Build history of the part. All positions in model axes, mm. Face numbers are marked on the shaded views. A direction names the side the tool comes from. Give positions to 0.01 mm unless a question says otherwise; leave off trailing zeros. Order: outer loops, then holes, each group sorted by start corner. A loop starts at its lowest first (then second) coordinate and runs counter-clockwise, first axis right, second up. Notation, with made-up numbers: (60, 41) - (69, 41) arc R18 cw to (69, 63) - close; hole circle Ø4 at (-25.5, 18.5). An arc over 180 degrees is marked (long way). Use a Markdown table: item, result.
from build123d import *

# Parameters (mm, degrees)
CROQUIS2_R              = 1.55
SALIENTE_EXTRUIR1_DEPTH = 5
REDONDEO9_R             = 5


with BuildPart() as part:
    # Croquis2 → Saliente-Extruir1 (new body)
    with BuildSketch(Plane(origin=(0, 0, 0), x_dir=(1, 0, 0), z_dir=(0, 1, 0))):
        Polygon((16, -17.5), (16, 17.5), (-16, 17.5), (-16, 8), (12, 8), (12, -8), (-16, -8), (-16, -17.5), align=None)
        with Locations(Location((-12.5, -12.5, 0), (0, 0, 270))):
            Circle(CROQUIS2_R, mode=Mode.SUBTRACT)
        with Locations(Location((12.5, -12.5, 0), (0, 0, 270))):
            Circle(CROQUIS2_R, mode=Mode.SUBTRACT)
        with Locations(Location((-12.5, 12.5, 0), (0, 0, 270))):
            Circle(CROQUIS2_R, mode=Mode.SUBTRACT)
        with Locations(Location((12.5, 12.5, 0), (0, 0, 270))):
            Circle(CROQUIS2_R, mode=Mode.SUBTRACT)
    extrude(amount=SALIENTE_EXTRUIR1_DEPTH)

    # Redondeo9
    # the kernel refuses this fillet: 5 mm, written as the material it adds along each edge
    with BuildSketch(Plane(origin=(12, 0, 8), x_dir=(0, 0, -1), z_dir=(0, 1, 0)), Plane(origin=(12, 0, -8), x_dir=(-1, 0, 0), z_dir=(0, 1, 0))) as redondeo9_piece_1:
        with BuildLine():
            CenterArc((REDONDEO9_R, REDONDEO9_R), REDONDEO9_R, 180, 90)
            Line((0, REDONDEO9_R), (0, 0))
            Line((0, 0), (REDONDEO9_R, 0))
        make_face()
    extrude(amount=5)
    # the kernel refuses this fillet: 5 mm, written as the material it takes off along each edge
    with BuildSketch(Plane(origin=(-16, -12.5, 8), x_dir=(0, 0, 1), z_dir=(0, 1, 0))) as redondeo9_2_piece_1:
        with BuildLine():
            CenterArc((REDONDEO9_R, REDONDEO9_R), REDONDEO9_R, 180, 90)
            Line((0, REDONDEO9_R), (0, 0))
            Line((0, 0), (REDONDEO9_R, 0))
        make_face()
    extrude(amount=30, mode=Mode.SUBTRACT)
    with BuildSketch(Plane(origin=(-16, -12.5, 17.5), x_dir=(0, 0, -1), z_dir=(0, 1, 0)), Plane(origin=(-16, -12.5, -17.5), x_dir=(1, 0, 0), z_dir=(0, 1, 0)), Plane(origin=(16, -12.5, -17.5), x_dir=(0, 0, 1), z_dir=(0, 1, 0)), Plane(origin=(-16, -12.5, -8), x_dir=(0, 0, -1), z_dir=(0, 1, 0)), Plane(origin=(16, -12.5, 17.5), x_dir=(-1, 0, 0), z_dir=(0, 1, 0))) as redondeo9_2_piece_2:
        with BuildLine():
            CenterArc((REDONDEO9_R, -REDONDEO9_R), REDONDEO9_R, 90, 90)
            Line((0, -REDONDEO9_R), (0, 0))
            Line((0, 0), (REDONDEO9_R, 0))
        make_face()
    extrude(amount=30, mode=Mode.SUBTRACT)


solid = part.part
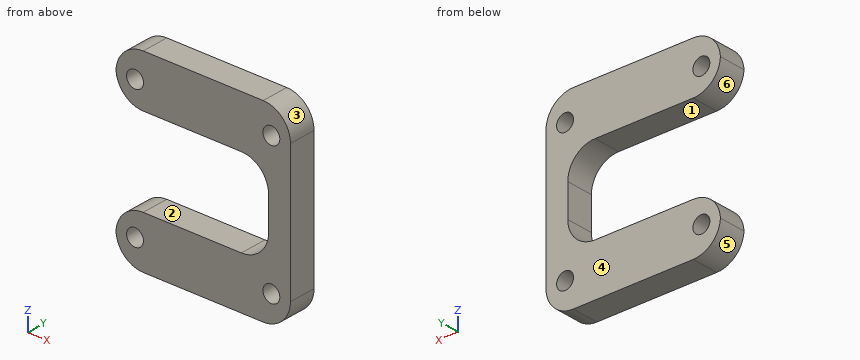
1) Wall check: line 1 (X direction, y = 3.85, z = 12.5); line 2 (Z direction, x = 3, y = 1.7); line 3 (Z direction, x = -11.5, y = 2.35). Give the ranges that are in metal, low to high. Write a range as from..to.
Computed:
| item | result |
|---|---|
| line 1 | x = -15.97..-14.05, -10.95..10.95, 14.05..16 |
| line 2 | z = -17.5..-8, 8..17.5 |
| line 3 | z = -17.47..-13.68, -11.32..-8.03, 8.03..11.32, 13.68..17.47 |
2) Slice it at D-D (z = 7). Write the cut outline in (x, y).
Computed:
| item | result |
|---|---|
| outline | (10, 0) - (16, 0) - (16, 5) - (10, 5) - close |
3) Slice it at C-C (x = -12.5). Write the cut outline in (y, z).
Computed:
| item | result |
|---|---|
| outline | (0, -17.27) - (5, -17.27) - (5, -14.05) - (0, -14.05) - close; (0, -10.95) - (5, -10.95) - (5, -8.23) - (0, -8.23) - close; (0, 8.23) - (5, 8.23) - (5, 10.95) - (0, 10.95) - close; (0, 14.05) - (5, 14.05) - (5, 17.27) - (0, 17.27) - close |
4) Two-plate mould, pull along Z, no slides. Class the marked faces 1, 2, 3 and 4: +Z half, -Z half, draft (parallel to the pull), parting line (faces both ways), or undercut.
Computed:
| item | result |
|---|---|
| face 1 | undercut |
| face 2 | undercut |
| face 3 | +Z half |
| face 4 | draft |
5) Tool access for the marked faces 5 and 6: list every direction of +Z, -Z, +X, -X, +Y, -Y with a clear straight run to the whole face (end or side of a thin tool).
Computed:
| item | result |
|---|---|
| face 5 | -Z, -X, +Y, -Y |
| face 6 | -X, +Y, -Y |
6) Slice it at B-B (x = 4). Write the cut outline in (y, z).
Computed:
| item | result |
|---|---|
| outline | (0, -17.5) - (5, -17.5) - (5, -8) - (0, -8) - close; (0, 8) - (5, 8) - (5, 17.5) - (0, 17.5) - close |
7) Slice it at A-A (y = 3.65). Write the cut outline in (x, z).
Computed:
| item | result |
|---|---|
| outline | (-15.99, -12.75) arc R5 ccw to (-11, -17.5) - (11, -17.5) arc R5 ccw to (16, -12.5) - (16, 12.5) arc R5 ccw to (11, 17.5) - (-11, 17.5) arc R5 ccw to (-15.99, 12.75) arc R5 ccw to (-11, 8) - (7, 8) arc R5 cw to (12, 3) - (12, -3) arc R5 cw to (7, -8) - (-11, -8) arc R5 ccw to start; hole circle Ø3.1 at (-12.5, -12.5); hole circle Ø3.1 at (-12.5, 12.5); hole circle Ø3.1 at (12.5, -12.5); hole circle Ø3.1 at (12.5, 12.5) |
